Solid Edge part; units mm, degrees
sketch "Sketch1" plane through (0, 0, 0) normal (0, 0, 1) x (1, 0, 0)
  circle A0 centre (0, 0) radius 4
  line L0 (-3.826, 6.6268) -> (-7.652, 0)
  line L1 (-7.652, 0) -> (-3.826, -6.6268)
  line L2 (-3.826, -6.6268) -> (3.826, -6.6268)
  line L3 (3.826, -6.6268) -> (7.652, 0)
  line L4 (7.652, 0) -> (3.826, 6.6268)
  line L5 (3.826, 6.6268) -> (-3.826, 6.6268)
extrude "Protrusion1" add sketch "Sketch1" along normal blind 5.356
cosmetic_thread "Thread1"
properties material "Steel"
Can you work these out from the model? Positions are in its coordinate system, mm. Coordinates: 2 decimals unless noted, no trailing zeros. Loops run counter-clockwise (first coordinate to the right, second up) from the corner with the lowest first, then second, coordinate; pieces in that order, holes last. Notation, with made-up numbers: (84.5, 8.5) - (100.5, 8.5) arc R27 ccw to (100.5, 35.5) - close; hole circle Ø3 at (87, 17.25). An arc over 180 degrees is marked (long way). Answer as CSV lines item,"result". Start each with the question number.
1) Suppose I cut it at C-C (y = 2.25). Please give me the cut outline in (x, z), plus the area to 3 significant figures.
2) I need wall thicknesses on line 1 (Y direction, x = 0, z = 3.3); line 2 (X direction, y = 2.5, z = 3.9); line 3 (X direction, y = 2.25, z = 4). Which ranges of each line are inside material? Lowest first, please. Write a range as from..to.
3) Suppose I cut it at B-B (z = 3.9). Please give me the cut outline in (x, y).
4) For pin 1 (1 mm diameter, centred on y = 1, z = 4.5, fed in from -X), with a flat end and sliding along its axis, tell me the tip position at first contact or that it passes through.
5) Suppose I cut it at D-D (x = 6.5). Please give me the cut outline in (y, z).
6) Suppose I cut it at A-A (x = 0). Please give me the cut outline in (y, z).
Check result:
1,outline,"(-6.35, 0) - (-3.31, 0) - (-3.31, 5.36) - (-6.35, 5.36) - close; (3.31, 0) - (6.35, 0) - (6.35, 5.36) - (3.31, 5.36) - close"
1,area,"32.6 mm²"
2,line 1,"y = -6.63..-4, 4..6.63"
2,line 2,"x = -6.21..-3.12, 3.12..6.21"
2,line 3,"x = -6.35..-3.31, 3.31..6.35"
3,outline,"(-7.65, 0) - (-3.83, -6.63) - (3.83, -6.63) - (7.65, 0) - (3.83, 6.63) - (-3.83, 6.63) - close; hole circle Ø8 at (0, 0)"
4,pin 1,"stops at x = -7.36"
5,outline,"(-2, 0) - (2, 0) - (2, 5.36) - (-2, 5.36) - close"
6,outline,"(-6.63, 0) - (-4, 0) - (-4, 5.36) - (-6.63, 5.36) - close; (4, 0) - (6.63, 0) - (6.63, 5.36) - (4, 5.36) - close"
